Verification items for the finished model (mm, model axes). Give positions to 0.01 mm unless a question says otherwise; leave off trailing zeros. Order: outer loops, then holes, each group sorted by start corner. A loop starts at its lowest first (then second) coordinate and runs counter-clockwise, first axis right, second up.
(1) Mould release check, pull along Y, two halves, no side actions. Record for faces 1 (the face through (18.25, 0.08, 2.28)), 2 (the face through (32.75, -0.06, 2.22)), 3 (the face through (15, 2, 0)): pulls with the +Y half, pulls with the -Y half, needs draft (parallel to the pull), parting line crosses it, or undercut.
(2) Gauge pin test, flat ends, axial feed: pin 1 (3 mm diameter, centred on x = 25, y = 0, fed in from -Z); pin 2 (1 mm diameter, centred on y = 2, z = 2.5, fed in from -X). Record the tip position at first contact, or that the pin passes through.
(3) Sectioned sample at A-A on y = 0. Count the separate pieces of the cut face and the enclosed holes in it, plus the area to 3 significant figures.
(4) Sectioned sample at D-D on x = 6. Record the cut outline in (y, z).
(5) Sectioned sample at C-C on x = 20. Record the cut outline in (y, z), plus the area to 3 significant figures.
(6) Sectioned sample at B-B on z = 3.9. Record the cut outline in (x, y), plus the area to 3 significant figures.
(7) Scan lines: L1, parallel to Y at x = 25, z = 1.6; L2, parallel to X at y = 1.8, z = 2.05. Record each from-to range of solid material in increasing order.
```python
from build123d import *

# Parameters (mm, degrees)
PAD_DEPTH           = 4.5
SKETCH001_R         = 1.75
POCKET_DEPTH        = 4.501
LINEARPATTERN_COUNT = 7
LINEARPATTERN_PITCH = 5


with BuildPart() as part:
    # Sketch → Pad (new body)
    with BuildSketch(Plane.XY):
        with BuildLine():
            ThreePointArc((1.4e-05, 2.75), (-2.75, 7e-06), (0, -2.75))
            Line((0, -2.75), (30, -2.75))
            ThreePointArc((30, -2.75), (32.75, -7e-06), (30.000014, 2.75))
            Line((1.4e-05, 2.75), (30.000014, 2.75))
        make_face()
    extrude(amount=PAD_DEPTH)

    # Sketch001 → Pocket (cut, through all)
    with BuildSketch(Plane.XY.offset(4.5)):
        Circle(SKETCH001_R)
    pocket = extrude(amount=-POCKET_DEPTH, mode=Mode.SUBTRACT)

    # LinearPattern: Pocket ×7
    with Locations(*[(i * LINEARPATTERN_PITCH, 0, 0) for i in range(1, LINEARPATTERN_COUNT)]):
        add(pocket, mode=Mode.SUBTRACT)


solid = part.part
```
Ans:
1. face 1: undercut
1. face 2: parting line crosses it
1. face 3: needs draft
2. pin 1: passes through
2. pin 2: stops at x = -2.3
3. separate pieces: 8
3. enclosed holes: 0
3. area: 49.5 mm2
4. outline: (-2.75, 0) - (-1.44, 0) - (-1.44, 4.5) - (-2.75, 4.5) - close; (1.44, 0) - (2.75, 0) - (2.75, 4.5) - (1.44, 4.5) - close
5. outline: (-2.75, 0) - (-1.75, 0) - (-1.75, 4.5) - (-2.75, 4.5) - close; (1.75, 0) - (2.75, 0) - (2.75, 4.5) - (1.75, 4.5) - close
5. area: 9.00 mm2
6. outline: (0, -2.75) - (30, -2.75) arc R2.75 ccw to (30, 2.75) - (0, 2.75) arc R2.75 ccw to start; hole circle Ø3.5 at (0, 0); hole circle Ø3.5 at (5, 0); hole circle Ø3.5 at (10, 0); hole circle Ø3.5 at (15, 0); hole circle Ø3.5 at (20, 0); hole circle Ø3.5 at (25, 0); hole circle Ø3.5 at (30, 0)
6. area: 121 mm2
7. L1: y = -2.75 to -1.75, 1.75 to 2.75
7. L2: x = -2.08 to 32.08
